from build123d import *

# Parameters (mm, degrees)
F0_R     = 14.2875
F1_DEPTH = 64.135
F4_DEPTH = 30.48
F6_R     = 10.8050815028
F7_DEPTH = 19.05
F5_R     = 10.795
F8_DEPTH = 19.05
F2_R     = 10.795
F9_DEPTH = 19.05


with BuildPart() as f1:
    # F0 (on Front) → F1 (new body)
    with BuildSketch(Plane.XZ):
        Circle(F0_R)
    extrude(amount=F1_DEPTH)

    # F3 (on Top) → F4 (join)
    with BuildSketch(Plane.XY):
        with BuildLine():
            ThreePointArc((0, -45.4052215051), (10.1027881362, -41.2205096413), (14.2875, -31.1177215051))
            ThreePointArc((14.2875, -31.1177215051), (-10.1027881362, -21.0149333689), (0, -45.4052215051))
        make_face()
    extrude(amount=F4_DEPTH)

    # F6 (on face) → F7 (cut)
    with BuildSketch(Plane(origin=(0, 0, 0), x_dir=(-1, 0, 0), z_dir=(0, 1, 0))):
        Circle(F6_R)
    extrude(amount=-F7_DEPTH, mode=Mode.SUBTRACT)

    # F5 (on face) → F8 (cut)
    with BuildSketch(Plane.XY.offset(30.48)):
        with Locations((0, -31.1177215051)):
            Circle(F5_R)
    extrude(amount=-F8_DEPTH, mode=Mode.SUBTRACT)

    # F2 (on face) → F9 (cut)
    with BuildSketch(Plane.XZ.offset(64.135)):
        Circle(F2_R)
    extrude(amount=-F9_DEPTH, mode=Mode.SUBTRACT)


solid = f1.part
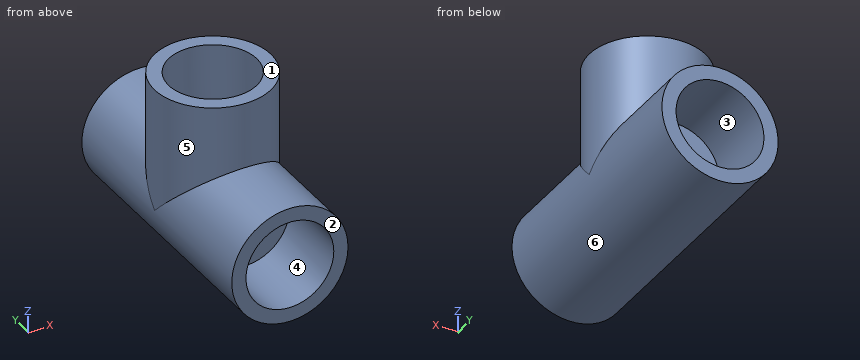
Geometry check sheet. Reference: the model listing, model coordinates, mm. Face numbers are marked on the shaded views. A direction names the side the tool comes from. Give positions to 0.01 mm unless a question says otherwise; leave off trailing zeros. Loops run counter-clockwise (first coordinate to the right, second up) from the corner with the lowest first, then second, coordinate; pieces in that order, holes last. Notation, with made-up numbers: (21.5, 41) -> (60.5, 41) arc R18 ccw to (60.5, 72) -> close; hole circle Ø10 at (70.5, 20). An arc over 180 degrees is marked (long way). Answer in a Markdown table with one row per item. Add a question column.
1) Cross-section at C-C on z = -5. Record the boundary of the cut face in (x, y) (3 decimals).
2) Cross-section at B-B on y = -10.5. Record the boundary of the cut face in (x, z) (1 decimal).
3) Draft check along Z on the marked faces 1, 2 and 3. Enter one of: pulls with the +Z half, pulls with the -Z half, needs draft (parallel to the pull), parting line crosses it, or undercut.
4) Set-up check for the marked faces 4, 5 and 6: record each of +Z, -Z, +X, -X, +Y, -Y from which the full face is reachable in a straight line by a thin tool's end or side.
5) Gauge pin test, flat ends, axial feed: P1, Ø3, axis at x = -5.5, y = -26, coming from the +Z side; P2, Ø5, axis at y = -54.5, z = -6.5, coming from the +X side; P3, Ø13, axis at x = 0, z = 0, coming from the -Y side (3 decimals). Record the tip position at first contact, or that the pin passes through.
6) Material ranges on probe 1 along Z at (x, y) = (0, -49.5) (1 decimal); probe 2 along Y at (x, z) = (-2, 2.5) (3 decimals); probe 3 along Z at (x, y) = (-7.75, -8), recorded low to high. Write a range as from..to.
7) Cross-section at D-D on y = -40.5. Record the boundary of the cut face in (x, z) (1 decimal).
Outcome:
| question | item | result |
|---|---|---|
| 1 | outline | (-13.384, -64.135) -> (-9.567, -64.135) -> (-9.567, -45.085) -> (9.567, -45.085) -> (9.567, -64.135) -> (13.384, -64.135) -> (13.384, 0) -> (9.579, 0) -> (9.579, -19.05) -> (-9.579, -19.05) -> (-9.579, 0) -> (-13.384, 0) -> close |
| 2 | outline | circle Ø28.6 at (0, 0); hole circle Ø21.6 at (0, 0) |
| 3 | face 1 | pulls with the +Z half |
| 3 | face 2 | needs draft |
| 3 | face 3 | undercut |
| 4 | face 4 | -Y |
| 4 | face 5 | +Z |
| 4 | face 6 | none |
| 5 | P1 | stops at z = 11.43 |
| 5 | P2 | stops at x = 13.72 |
| 5 | P3 | stops at y = -45.085 |
| 6 | probe 1 | z = -14.3..-10.8, 10.8..14.3 |
| 6 | probe 2 | y = -45.085..-19.05 |
| 6 | probe 3 | z = -12..-7.53, 7.53..12 |
| 7 | outline | (-10.8, 9.4) arc R14.3 ccw (long way) to (10.8, 9.4) -> (10.8, 30.5) -> (5.3, 30.5) -> (5.3, 11.4) -> (-5.3, 11.4) -> (-5.3, 30.5) -> (-10.8, 30.5) -> close |
